Here's the drawing with two shaded views (mm, measured from the low corner). I have some questions. A direction names the side the tool comes from. Coordinates: 2 decimals unless noted, no trailing zeros. Write each loop counter-clockwise with the first axis right and the second up, starting at its lowest first coordinate (ties: lowest second). Pieces come first, ordered by that corner, then holes.
Item 1: If we section it at A-A (z = 25): Please give me the cut outline in (x, y).
Item 2: If we section it at C-C (x = 28): Count the separate pieces of the cut face and the enclosed holes in it, then the cut area to 3 significant figures.
Item 3: I'm going to push flat-ended pins straight in: pin 1 Ø5.5 at (x, y) = (28, 25) entering from +Z; pin 2 Ø6 at (x, z) = (26, 41.5) entering from -Y; pin 3 Ø7.5 at (x, z) = (6, 25) entering from -Y. Where does each tip first touch, or does it pass through?
Item 4: If I drill on line 1 (X direction, y = 44, z = 25); line 2 (X direction, y = 36, z = 25); line 3 (Y direction, x = 7, z = 5.75), over which ranges is the centre line in solid material (lowest first)?
Item 5: If we section it at B-B (y = 25): Please give me the cut outline in (x, z), then the cut area to 3 significant figures.
Item 6: For the marked faces 1, 2, 3, 4 and 5, which set-ups out of +Z, -Z, +X, -X, +Y, -Y let a thin tool reach every point of the face, with its end or its side?
Item 7: We'd pull the mould along X, two halves only. Please class the marked faces 6, 7 and 8: +X half, -X half, draft (parallel to the pull), parting line (faces both ways), or undercut.
Item 8: If we section it at D-D (x = 18): Please give me the cut outline in (y, z), then the cut area to 3 significant figures.
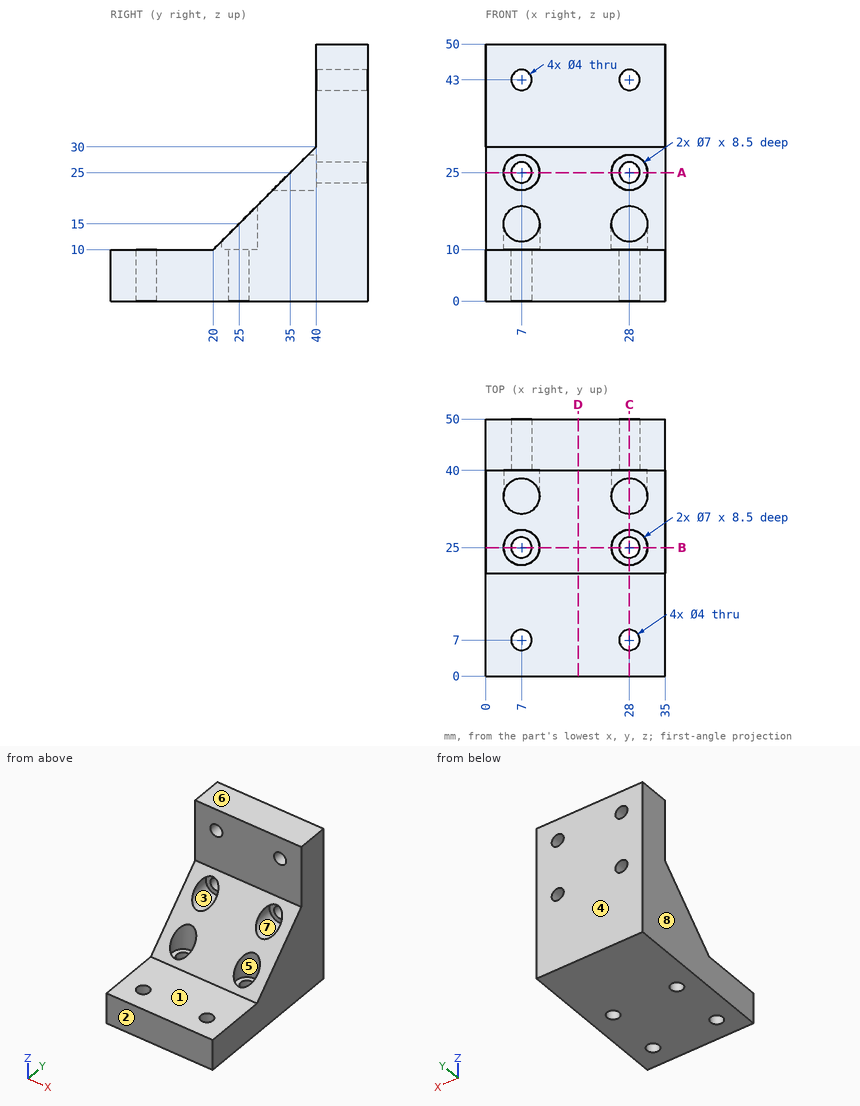
Answer list:
1. outline: (0, 35) - (3.5, 35) - (3.5, 40) - (5, 40) - (5, 50) - (0, 50) - close; (9, 40) - (10.5, 40) - (10.5, 35) - (24.5, 35) - (24.5, 40) - (26, 40) - (26, 50) - (9, 50) - close; (30, 40) - (31.5, 40) - (31.5, 35) - (35, 35) - (35, 50) - (30, 50) - close
2. separate pieces: 5
2. enclosed holes: 0
2. area: 870 mm2
3. pin 1: stops at z = 10
3. pin 2: stops at y = 40
3. pin 3: stops at y = 31.25
4. line 1: x = 0 to 5, 9 to 26, 30 to 35
4. line 2: x = 0 to 3.5, 10.5 to 24.5, 31.5 to 35
4. line 3: y = 0 to 5, 9 to 23, 27 to 50
5. outline: (0, 0) - (5, 0) - (5, 10) - (3.5, 10) - (3.5, 15) - (0, 15) - close; (9, 0) - (26, 0) - (26, 10) - (24.5, 10) - (24.5, 15) - (10.5, 15) - (10.5, 10) - (9, 10) - close; (30, 0) - (35, 0) - (35, 15) - (31.5, 15) - (31.5, 10) - (30, 10) - close
5. area: 375 mm2
6. face 1: +Z, +X, -X, -Y
6. face 2: +Z, -Z, +X, -X, -Y
6. face 3: -Y
6. face 4: +Z, -Z, +X, -X, +Y
6. face 5: +Z
7. face 6: draft
7. face 7: undercut
7. face 8: -X half
8. outline: (0, 0) - (50, 0) - (50, 50) - (40, 50) - (40, 30) - (20, 10) - (0, 10) - close
8. area: 1,100 mm2
